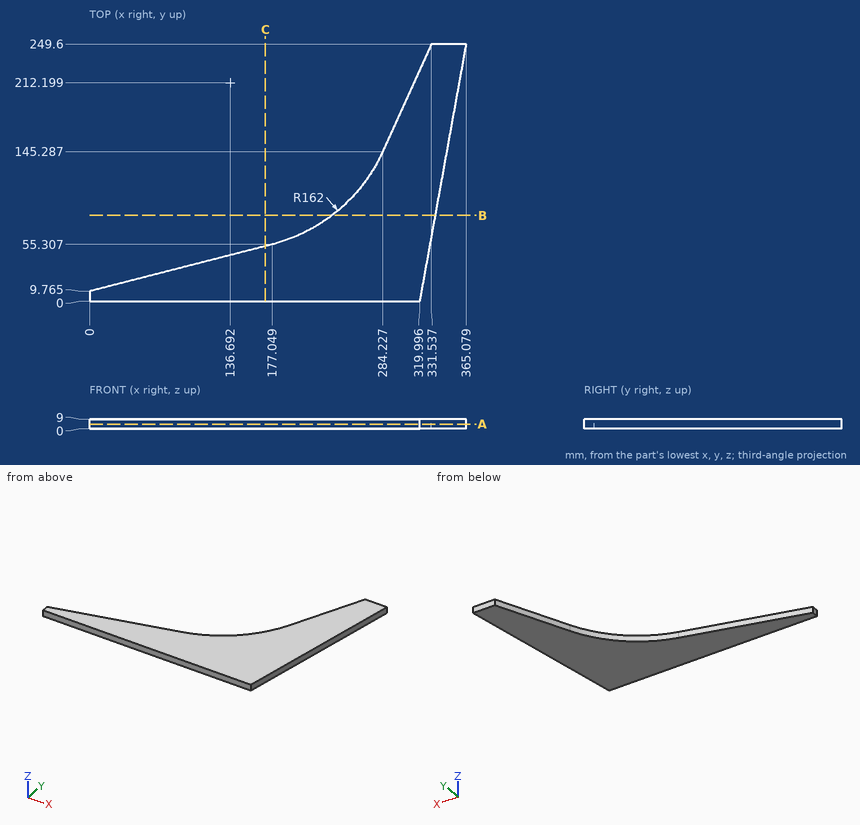
Geometry: see drawing. Coordinates: mm, zero at the bounding-box minimum. Give positions to 0.01 mm unless a question says otherwise; leave off trailing zeros. Loops run counter-clockwise (first coordinate to the right, second up) from the corner with the lowest first, then second, coordinate; pieces in that order, holes last. Notation, with made-up numbers: (16, 32.5) -> (38, 32.5) arc R23 cw to (38, 50.5) -> close; hole circle Ø9 at (11, 42). An arc over 180 degrees is marked (long way). Answer as a JSON object with one key per item and string values. Group by question number.
Item 1: Line query: probe 1 along Y at (x, z) = (145, 8); probe 2 along Y at (x, z) = (305.5, 2) (1 decimal); probe 3 along X at (y, z) = (63, 2) (1 decimal). Output: solid intervals per line, ascending.
Item 2: Cut plane A-A, the plane z = 4.5. Return the cut outline in (x, y) (1 decimal), and give its area (3 significant figures).
Item 3: Cut plane B-B, the plane y = 83.5. Return the cut outline in (x, z).
Item 4: Pin query (flat end, axial travel): P1, Ø12, axis at x = 204, y = 62.5, coming from the -Z side; P2, Ø1.5, axis at x = 244, z = 1.5, coming from the +Y side (1 decimal); P3, Ø5, axis at y = 82, z = 2, coming from the -X side (1 decimal); P4, Ø2, axis at y = 218.5, z = 6.5, coming from the -X side. Return the tip coordinate at first contact, or that it passes through.
Item 5: Cut plane C-C, the plane x = 170.5. Return the cut outline in (y, z).
Checks:
{
 "1": {"probe 1": "y = 0 to 47.06", "probe 2": "y = 0 to 192.2", "probe 3": "x = 199.8 to 331.4"},
 "2": {"outline": "(0, 0) -> (320, 0) -> (365.1, 249.6) -> (331.5, 249.6) -> (284.2, 145.3) arc R162 cw to (177, 55.3) -> (0, 9.8) -> close", "area": "27,100 mm²"},
 "3": {"outline": "(235.08, 0) -> (335.08, 0) -> (335.08, 9) -> (235.08, 9) -> close"},
 "4": {"P1": "stops at z = 0", "P2": "stops at y = 91.5", "P3": "stops at x = 229.6", "P4": "stops at x = 316.98"},
 "5": {"outline": "(0, 0) -> (53.62, 0) -> (53.62, 9) -> (0, 9) -> close"}
}
